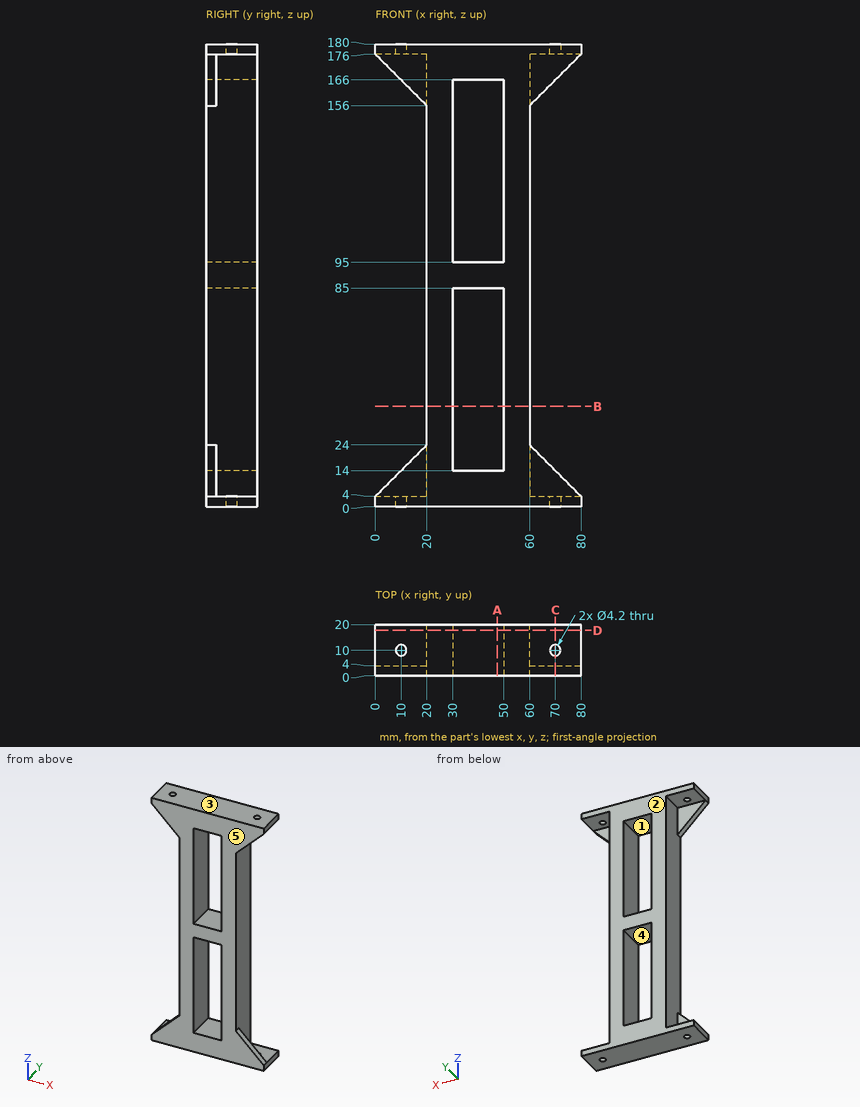
The drawing under review shows one solid part. Ordinate dimensions are in mm from its lowest x, y, z. A direction names the side the tool comes from. Coordinates: 2 decimals unless noted, no trailing zeros. Write each loop counter-clockwise with the first axis right and the second up, starting at its lowest first coordinate (ties: lowest second). Pieces come first, ordered by that corner, then holes. Notation, with made-up numbers: (77, 9) - (84, 9) arc R12 ccw to (84, 21) - close; hole circle Ø4 at (-0.75, 40.25). An arc over 180 degrees is marked (long way). Answer as CSV lines item,"result".
(1) For line 1 along Z through (x, y) = (39, 3.5); line 2 along X through (y, z) = (8.75, 117); line 3 along Z through (x, y) = (65, 6.25), list the stretches that pass through material, from the lowest coordinate up. Write a range as [from, to].
Data:
line 1,"z = [0, 14], [85, 95], [166, 180]"
line 2,"x = [20, 30], [50, 60]"
line 3,"z = [0, 4], [176, 180]"
(2) We need section B-B (z = 39). Give the boundary of the cut face in (x, y).
Data:
outline,"(20, 0) - (30, 0) - (30, 20) - (20, 20) - close; (50, 0) - (60, 0) - (60, 20) - (50, 20) - close"
(3) Tool access review of the marked faces 1 and 2: name each direction out of +Z, -Z, +X, -X, +Y, -Y from which nothing blocks a thin tool from reaching the whole face with its end or side.
Data:
face 1,"+Y, -Y"
face 2,"+Z, -Z, +X, -X, +Y"
(4) We need section A-A (x = 47.5). Give the boundary of the cut face in (y, z).
Data:
outline,"(0, 0) - (20, 0) - (20, 14) - (0, 14) - close; (0, 85) - (20, 85) - (20, 95) - (0, 95) - close; (0, 166) - (20, 166) - (20, 180) - (0, 180) - close"
(5) Mouldability with a two-part tool opening along Z and no side actions: class the marked faces 3, 4 and 5 as pulls with the +Z half, pulls with the -Z half, needs draft (parallel to the pull), parting line crosses it, or undercut.
Data:
face 3,"pulls with the +Z half"
face 4,"undercut"
face 5,"needs draft"
(6) We need section D-D (y = 17.75). Give the boundary of the cut face in (x, z), plus the area to 3 significant figures.
Data:
outline,"(0, 0) - (80, 0) - (80, 4) - (60, 4) - (60, 176) - (80, 176) - (80, 180) - (0, 180) - (0, 176) - (20, 176) - (20, 4) - (0, 4) - close; hole (30, 14) - (50, 14) - (50, 85) - (30, 85) - close; hole (30, 95) - (50, 95) - (50, 166) - (30, 166) - close"
area,"4,680 mm2"
(7) Clearance check with flat-ended pins moving along their axes: pin 1 Ø12 at (x, y) = (47, 15) entering from -Z; pin 2 Ø3 at (y, z) = (7, 122) entering from +X; pin 3 Ø10 at (x, z) = (12, 170.5) entering from +Y; pin 4 Ø4 at (x, y) = (70, 10) entering from -Z. State where each tip first meets the part, or that it passes through.
Data:
pin 1,"stops at z = 0"
pin 2,"stops at x = 60"
pin 3,"stops at y = 4"
pin 4,"passes through"
(8) We need section C-C (x = 70). Give the boundary of the cut face in (y, z).
Data:
outline,"(0, 0) - (7.9, 0) - (7.9, 4) - (4, 4) - (4, 14) - (0, 14) - close; (0, 166) - (4, 166) - (4, 176) - (7.9, 176) - (7.9, 180) - (0, 180) - close; (12.1, 0) - (20, 0) - (20, 4) - (12.1, 4) - close; (12.1, 176) - (20, 176) - (20, 180) - (12.1, 180) - close"
